Verification items for the finished model (mm, model axes). A direction names the side the tool comes from. Coordinates: 2 decimals unless noted, no trailing zeros. Loops run counter-clockwise (first coordinate to the right, second up) from the corner with the lowest first, then second, coordinate; pieces in that order, holes last. Notation, with made-up numbers: (10, -8) -> (40, -8) arc R13 cw to (40, 14) -> close; hole circle Ø9 at (-4, -11). An arc over 180 degrees is marked (long way). Write item = value, one per line.
```python
from build123d import *

# Parameters (mm, degrees)
SKETCH1_W                      = 69.85
SKETCH1_H                      = 50.8
BOSS_EXTRUDE1_DEPTH            = 10
SKETCH2_R                      = 15.875
CUT_EXTRUDE1_DEPTH             = 11
M5X0_8_TAPPED_HOLE1_D          = 4.2
CBORE_FOR_M6_SHCS1_D           = 6.4
CBORE_FOR_M6_SHCS1_CBORE_D     = 10.1
CBORE_FOR_M6_SHCS1_CBORE_DEPTH = 6
MIRROR2_COPY_1_D               = 4.2
MIRROR2_COPY_2_D               = 6.4
MIRROR2_COPY_2_CBORE_D         = 10.1
MIRROR2_COPY_2_CBORE_DEPTH     = 6
SKETCH7_R                      = 18.25625
SKETCH7_R_2                    = 15.875
BOSS_EXTRUDE2_DEPTH            = 33.02
SKETCH8_R                      = 18.85315
SKETCH8_R_2                    = 16.66875
CUT_EXTRUDE2_DEPTH             = 1.3208
SKETCH9_W                      = 2.4892
SKETCH9_H                      = 1.2954


with BuildPart() as part:
    # Sketch1 → Boss-Extrude1 (new body)
    with BuildSketch(Plane.XY):
        Rectangle(SKETCH1_W, SKETCH1_H)
    extrude(amount=BOSS_EXTRUDE1_DEPTH)

    # Sketch2 → Cut-Extrude1 (cut, through all)
    with BuildSketch(Plane.XY.offset(10)):
        Circle(SKETCH2_R)
    extrude(amount=-CUT_EXTRUDE1_DEPTH, mode=Mode.SUBTRACT)

    # M5x0.8 Tapped Hole1 (through all)
    with Locations(Plane.XY.offset(10)):
        with Locations((30, 19.999999878)):
            m5x0_8_tapped_hole1 = Hole(M5X0_8_TAPPED_HOLE1_D / 2)

    # CBORE for M6 SHCS1 (through all)
    with Locations(Plane(origin=(0, 0, 0), x_dir=(-1, 0, 0), z_dir=(0, 0, -1))):
        with Locations((-15, 20)):
            cbore_for_m6_shcs1 = CounterBoreHole(CBORE_FOR_M6_SHCS1_D / 2, CBORE_FOR_M6_SHCS1_CBORE_D / 2, CBORE_FOR_M6_SHCS1_CBORE_DEPTH)

    # Mirror1: M5x0.8 Tapped Hole1, CBORE for M6 SHCS1 across plane
    add(m5x0_8_tapped_hole1.mirror(Plane.ZX), mode=Mode.SUBTRACT)
    add(cbore_for_m6_shcs1.mirror(Plane.ZX), mode=Mode.SUBTRACT)

    # Mirror2: M5x0.8 Tapped Hole1, CBORE for M6 SHCS1 across plane
    add(m5x0_8_tapped_hole1.mirror(Plane(origin=(0, 0, 0), x_dir=(0, 0, 1), z_dir=(1, 0, 0))), mode=Mode.SUBTRACT)
    add(cbore_for_m6_shcs1.mirror(Plane(origin=(0, 0, 0), x_dir=(0, 0, 1), z_dir=(1, 0, 0))), mode=Mode.SUBTRACT)

    # Mirror2 copy 1 (through all)
    with Locations(Plane(origin=(0, 0, 10), x_dir=(-1, 0, 0), z_dir=(0, 0, 1))):
        with Locations((30, 19.999999878)):
            Hole(MIRROR2_COPY_1_D / 2)

    # Mirror2 copy 2 (through all)
    with Locations(Plane(origin=(0, 0, 0), x_dir=(1, 0, 0), z_dir=(0, 0, -1))):
        with Locations((-15, 20)):
            CounterBoreHole(MIRROR2_COPY_2_D / 2, MIRROR2_COPY_2_CBORE_D / 2, MIRROR2_COPY_2_CBORE_DEPTH)

    # Sketch7 → Boss-Extrude2 (add)
    with BuildSketch(Plane.XY.offset(10)):
        Circle(SKETCH7_R)
        Circle(SKETCH7_R_2, mode=Mode.SUBTRACT)
    extrude(amount=BOSS_EXTRUDE2_DEPTH)

    # Sketch8 → Cut-Extrude2 (cut)
    with BuildSketch(Plane(origin=(0, 0, 0), x_dir=(-1, 0, 0), z_dir=(0, 0, -1))):
        Circle(SKETCH8_R)
        Circle(SKETCH8_R_2, mode=Mode.SUBTRACT)
    extrude(amount=-CUT_EXTRUDE2_DEPTH, mode=Mode.SUBTRACT)

    # Sketch9 → Cut-Revolve1 (revolve, cut)
    with BuildSketch(Plane(origin=(0, 0, 0), x_dir=(0, 0, -1), z_dir=(1, 0, 0))):
        with Locations((-40.1879, -17.85874)):
            Rectangle(SKETCH9_W, SKETCH9_H)
    revolve(axis=Axis((0, 0, -4.391211434), (0, 0, 1)), mode=Mode.SUBTRACT)


solid = part.part
```
1) Tool access check on faces 4 (the face through (14.306, 16.876, 8.028)), 5 (the face through (17.413, 5.484, 42.215)), 6 (the face through (12.3, 12.3, 41.432)), 7 (the face through (-12.29, -24.26, 2.96)). Record the directions out of +Z, -Z, +X, -X, +Y, -Y that give a thin tool (end or side, any length) a straight path to the whole face; none if there is none.
Ans:
face_4 = +Z, -Z
face_5 = +Z
face_6 = none
face_7 = -Z
2) Sectioned sample at A-A, the plane y = 0. Record the cut outline in (x, z) (1 decimal).
Ans:
outline = (-34.9, 0) -> (-18.9, 0) -> (-18.9, 1.3) -> (-16.7, 1.3) -> (-16.7, 0) -> (-15.9, 0) -> (-15.9, 43) -> (-18.3, 43) -> (-18.3, 41.4) -> (-17.2, 41.4) -> (-17.2, 38.9) -> (-18.3, 38.9) -> (-18.3, 10) -> (-34.9, 10) -> close; (15.9, 0) -> (16.7, 0) -> (16.7, 1.3) -> (18.9, 1.3) -> (18.9, 0) -> (34.9, 0) -> (34.9, 10) -> (18.3, 10) -> (18.3, 38.9) -> (17.2, 38.9) -> (17.2, 41.4) -> (18.3, 41.4) -> (18.3, 43) -> (15.9, 43) -> close
3) Sectioned sample at C-C, the plane z = 5. Count the separate pieces of the cut face and the enclosed holes in it, plus the area to 3 significant figures.
Ans:
separate_pieces = 1
enclosed_holes = 9
area = 2,380 mm2
4) Depth check by flat-ended pin: pin 1 Ø8 at (x, z) = (6, 29.5) entering from -Y; pin 2 Ø5 at (x, y) = (-15.5, 21) entering from -Z; pin 3 Ø5.5 at (x, y) = (-30, 20) entering from -Z; pin 4 Ø12 at (y, z) = (-12.5, 24.5) entering from +X. Enter the tip coordinate at first touch or a pass-through.
Ans:
pin_1 = -18.15
pin_2 = 6
pin_3 = 0
pin_4 = 17.06
5) Sectioned sample at B-B, the plane x = -30. Record the cut outline in (y, z), plus the area to 3 significant figures.
Ans:
outline = (-25.4, 0) -> (-22.1, 0) -> (-22.1, 10) -> (-25.4, 10) -> close; (-17.9, 0) -> (17.9, 0) -> (17.9, 10) -> (-17.9, 10) -> close; (22.1, 0) -> (25.4, 0) -> (25.4, 10) -> (22.1, 10) -> close
area = 424 mm2
6) Material ranges on line 1 (Y direction, x = -30, z = 6.75); line 2 (Y direction, x = 0, z = 28) (3 decimals); line 3 (Y direction, x = -10.5, z = 17), recorded low to high.
Ans:
line_1 = -25.4 to -22.1, -17.9 to 17.9, 22.1 to 25.4
line_2 = -18.256 to -15.875, 15.875 to 18.256
line_3 = -14.93 to -11.91, 11.91 to 14.93
7) Release check for a two-part mould opening along Y. For faces 1 (the face through (12.3, 12.3, 38.943)), 2 (the face through (5.17, -16.416, 40.17)), 3 (the face through (0, -17, 1.321)) record: pulls with the +Y half, pulls with the -Y half, needs draft (parallel to the pull), parting line crosses it, or undercut.
Ans:
face_1 = needs draft
face_2 = parting line crosses it
face_3 = undercut
8) Sectioned sample at D-D, the plane y = 20. Record the cut outline in (x, z) (3 decimals).
Ans:
outline = (-34.925, 0) -> (-32.1, 0) -> (-32.1, 10) -> (-34.925, 10) -> close; (-27.9, 0) -> (-20.05, 0) -> (-20.05, 6) -> (-18.2, 6) -> (-18.2, 10) -> (-27.9, 10) -> close; (-11.8, 6) -> (-9.95, 6) -> (-9.95, 0) -> (9.95, 0) -> (9.95, 6) -> (11.8, 6) -> (11.8, 10) -> (-11.8, 10) -> close; (18.2, 6) -> (20.05, 6) -> (20.05, 0) -> (27.9, 0) -> (27.9, 10) -> (18.2, 10) -> close; (32.1, 0) -> (34.925, 0) -> (34.925, 10) -> (32.1, 10) -> close
